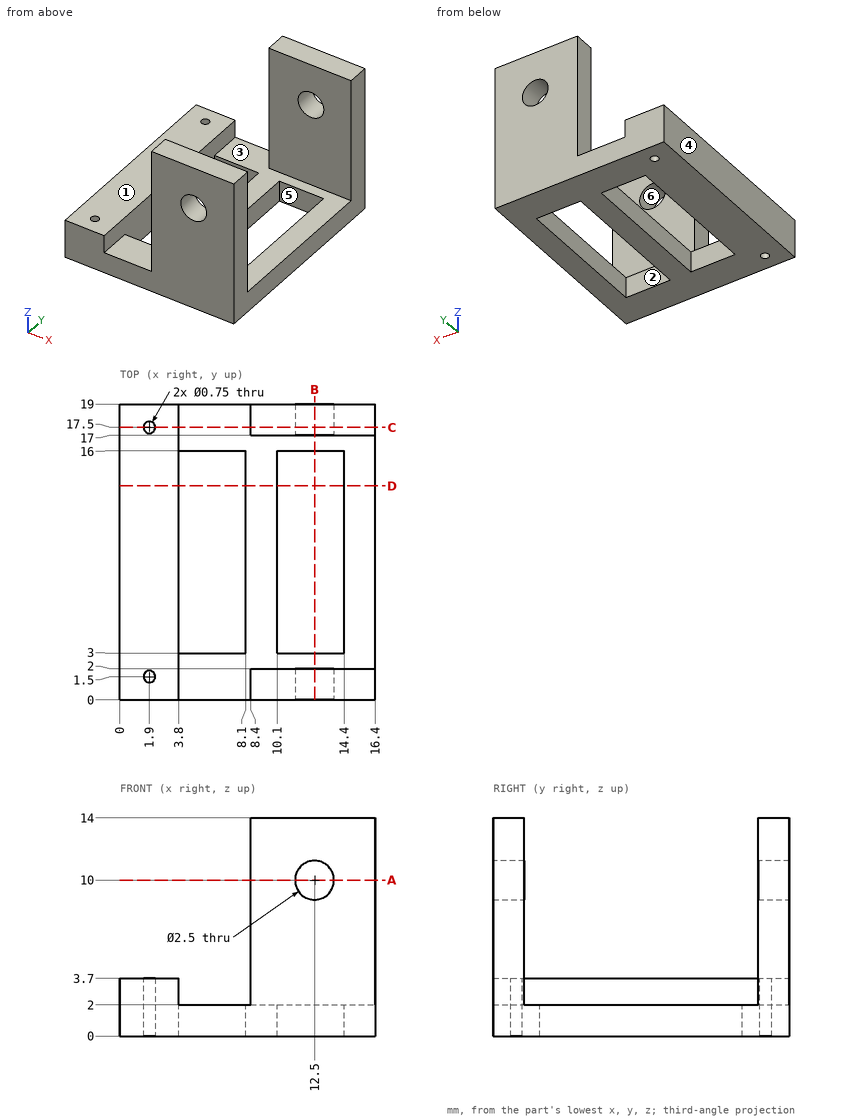
Print and shaded views of the part. All mm, measured from the part's lowest x, y and z. A direction names the side the tool comes from. Coordinates: 2 decimals unless noted, no trailing zeros. Order: outer loops, then holes, each group sorted by start corner. A loop starts at its lowest first (then second) coordinate and runs counter-clockwise, first axis right, second up. Notation, with made-up numbers: (26.5, 68) - (33.5, 68) arc R18 ccw to (33.5, 80) - close; hole circle Ø3 at (-34, -21.5). An arc over 180 degrees is marked (long way). Return JSON: item names as keys, results as strings. Group by question number.
Item 1: Cut at B-B (x = 12.5). List the corners of the cut face in (y, z).
Item 2: Which spindle directions (+Z, -Z, +X, -X, +Y, -Y) get a long thin tool onto all of the face, cutting with end or side? Do the marked faces 5 and 6. Say none if no direction does.
Item 3: Pull direction X, two halves, no side cores. Call the marked faces 1, 2, 3 and 4: pulls with the +X half, pulls with the -X half, needs draft (parallel to the pull), parting line crosses it, or undercut.
Item 4: Pin check, flat tip, straight feed: pin 1 (1.5 mm diameter, centred on y = 2.5, z = 12, fed in from -X). Stop position of the tip, or through.
Item 5: Drill centre lines: probe 1 along X at (y, z) = (14, 1); probe 2 along Y at (x, z) = (1.9, 2.95) (3 decimals); probe 3 along Y at (x, z) = (12, 1.25). Where is each one in solid material? Low to high. Write a range as from..to.
Item 6: Cut at A-A (z = 10). List the corners of the cut face in (x, y), plus the area to 3 significant figures.
Item 7: Cut at C-C (y = 17.5). List the corners of the cut face in (x, z) (3 decimals), plus the area to 3 significant figures.
Item 8: Cut at D-D (y = 13.75). List the corners of the cut face in (x, z).
Check values:
{
 "1": {"outline": "(0, 0) - (3, 0) - (3, 2) - (2, 2) - (2, 8.75) - (0, 8.75) - close; (0, 11.25) - (2, 11.25) - (2, 14) - (0, 14) - close; (16, 0) - (19, 0) - (19, 8.75) - (17, 8.75) - (17, 2) - (16, 2) - close; (17, 11.25) - (19, 11.25) - (19, 14) - (17, 14) - close"},
 "2": {"face 5": "+Z, -Z", "face 6": "+Y, -Y"},
 "3": {"face 1": "needs draft", "face 2": "undercut", "face 3": "undercut", "face 4": "pulls with the -X half"},
 "4": {"pin 1": "stops at x = 8.4"},
 "5": {"probe 1": "x = 0..3.8, 8.1..10.1, 14.4..16.4", "probe 2": "y = 0..1.125, 1.875..17.125, 17.875..19", "probe 3": "y = 0..3, 16..19"},
 "6": {"outline": "(8.4, 0) - (11.25, 0) - (11.25, 2) - (8.4, 2) - close; (8.4, 17) - (11.25, 17) - (11.25, 19) - (8.4, 19) - close; (13.75, 0) - (16.4, 0) - (16.4, 2) - (13.75, 2) - close; (13.75, 17) - (16.4, 17) - (16.4, 19) - (13.75, 19) - close", "area": "22.0 mm2"},
 "7": {"outline": "(0, 0) - (1.525, 0) - (1.525, 3.7) - (0, 3.7) - close; (2.275, 0) - (16.4, 0) - (16.4, 14) - (8.4, 14) - (8.4, 2) - (3.8, 2) - (3.8, 3.7) - (2.275, 3.7) - close; hole circle Ø2.5 at (12.5, 10)", "area": "128 mm2"},
 "8": {"outline": "(0, 0) - (3.8, 0) - (3.8, 3.7) - (0, 3.7) - close; (8.1, 0) - (10.1, 0) - (10.1, 2) - (8.1, 2) - close; (14.4, 0) - (16.4, 0) - (16.4, 2) - (14.4, 2) - close"}
}
